The listing builds one solid part. Answer for the finished solid, in the listing's coordinates (mm). A direction names the side the tool comes from. Give positions to 0.01 mm unless a question says otherwise; leave off trailing zeros. Order: outer loops, then holes, each group sorted by start corner. A loop starts at its lowest first (then second) coordinate and runs counter-clockwise, first axis right, second up.
```python
from build123d import *

# Parameters (mm, degrees)
SKETCH1_W                                = 65
SKETCH1_H                                = 38.1
SKETCH1_W_2                              = 41
SKETCH1_H_2                              = 21
BOSS_EXTRUDE1_DEPTH                      = 8
SKETCH2_W                                = 65
SKETCH2_H                                = 38.1
SKETCH2_W_2                              = 59
SKETCH2_H_2                              = 26.1
BOSS_EXTRUDE2_DEPTH                      = 15
F_5_32_0_15625_DIAMETER_HOLE1_D          = 3.96875
F_3_0MM_DOWEL_HOLE1_D                    = 3
F_3_0MM_DOWEL_HOLE1_DEPTH                = 6
CUT_EXTRUDE1_DEPTH                       = 2.25
MIRROR2_AT_THE_SECOND_PLANE_COPY_1_DEPTH = 2.25


with BuildPart() as part:
    # Sketch1 → Boss-Extrude1 (new body)
    with BuildSketch(Plane(origin=(0, 0, 0), x_dir=(0, 0, -1), z_dir=(1, 0, 0))):
        Rectangle(SKETCH1_W, SKETCH1_H)
        Rectangle(SKETCH1_W_2, SKETCH1_H_2, mode=Mode.SUBTRACT)
    extrude(amount=BOSS_EXTRUDE1_DEPTH)

    # Sketch2 → Boss-Extrude2 (add)
    with BuildSketch(Plane(origin=(8, 0, 0), x_dir=(0, 0, -1), z_dir=(1, 0, 0))):
        Rectangle(SKETCH2_W, SKETCH2_H)
        Rectangle(SKETCH2_W_2, SKETCH2_H_2, mode=Mode.SUBTRACT)
    extrude(amount=BOSS_EXTRUDE2_DEPTH)

    # 5/32 (0.15625) Diameter Hole1 (through all)
    with Locations(Plane.ZY):
        with Locations((-23.60854322, 5.122882485), (-23.749, -5.08), (23.749, -5.08), (23.749, 5.08)):
            Hole(F_5_32_0_15625_DIAMETER_HOLE1_D / 2)

    # Ø3.0mm Dowel Hole1
    with Locations(Plane(origin=(0, -13.05, 0), x_dir=(1, 0, 0), z_dir=(0, 1, 0))):
        with Locations((11.5, 25), (11.5, -25)):
            f_3_0mm_dowel_hole1 = Hole(F_3_0MM_DOWEL_HOLE1_D / 2, depth=F_3_0MM_DOWEL_HOLE1_DEPTH)

    # Mirror1: Ø3.0mm Dowel Hole1 across plane
    add(f_3_0mm_dowel_hole1.mirror(Plane.ZX), mode=Mode.SUBTRACT)

    # Sketch7 → Cut-Extrude1 (cut)
    with BuildSketch(Plane(origin=(0, -13.05, 0), x_dir=(1, 0, 0), z_dir=(0, 1, 0))):
        Polygon((8.775, -26.573279484), (11.5, -28.146558967), (14.225, -26.573279484), (14.225, -23.426720516), (11.5, -21.853441033), (8.775, -23.426720516), align=None)
    cut_extrude1 = extrude(amount=-CUT_EXTRUDE1_DEPTH, mode=Mode.SUBTRACT)

    # Mirror2: Cut-Extrude1 across plane
    add(cut_extrude1.mirror(Plane.ZX), mode=Mode.SUBTRACT)

    # Mirror2 at the second plane: Cut-Extrude1 across plane
    add(cut_extrude1.mirror(Plane.XY), mode=Mode.SUBTRACT)

    # Mirror2 at the second plane copy 1 sketc → Mirror2 at the second plane copy 1 (cut)
    with BuildSketch(Plane.XZ.offset(-13.05)):
        Polygon((8.775, -26.573279484), (11.5, -28.146558967), (14.225, -26.573279484), (14.225, -23.426720516), (11.5, -21.853441033), (8.775, -23.426720516), align=None)
    extrude(amount=-MIRROR2_AT_THE_SECOND_PLANE_COPY_1_DEPTH, mode=Mode.SUBTRACT)


solid = part.part
```
1) A tool of negligible diameter and unlimited length cuts with its end or side. For faces 1 (the flat face through (15, -13.05, 0)), 2 (the flat face through (13, 15.3, -26)), 3 (the flat face through (4, 0, -20.5)), from which of +Z, -Z, +X, -X, +Y, -Y can it reach the whole face along a straight path? Write none if from no direction.
Geometry says:
face 1: +X
face 2: none
face 3: +X, -X
2) Find section B-B (z = -17). Write down the section's boundary in (x, y), then the cut area to 3 significant figures.
Geometry says:
outline: (0, -19.05) - (23, -19.05) - (23, -13.05) - (8, -13.05) - (8, -10.5) - (0, -10.5) - close; (0, 10.5) - (8, 10.5) - (8, 13.05) - (23, 13.05) - (23, 19.05) - (0, 19.05) - close
area: 317 mm2
3) Find section A-A (y = 1). Write down the section's boundary in (x, z), then the cut area to 3 significant figures.
Geometry says:
outline: (0, -32.5) - (23, -32.5) - (23, -29.5) - (8, -29.5) - (8, -20.5) - (0, -20.5) - close; (0, 20.5) - (8, 20.5) - (8, 29.5) - (23, 29.5) - (23, 32.5) - (0, 32.5) - close
area: 282 mm2
4) Find section D-D (x = 19.5). Write down the section's boundary in (y, z), then the cut area to 3 significant figures.
Geometry says:
outline: (-19.05, -32.5) - (19.05, -32.5) - (19.05, 32.5) - (-19.05, 32.5) - close; hole (-13.05, -29.5) - (13.05, -29.5) - (13.05, 29.5) - (-13.05, 29.5) - close
area: 937 mm2
5) Straight lines are drawn through the part: probe 1 along Y at (x, z) = (8.25, -7); probe 2 along Y at (x, z) = (4.75, 9.5); probe 3 along Z at (x, y) = (11.5, -16.1). For each, find the intervals that lie inside material, in ascending order.
Geometry says:
probe 1: y = -19.05 to -13.05, 13.05 to 19.05
probe 2: y = -19.05 to -10.5, 10.5 to 19.05
probe 3: z = -32.5 to -26.5, -23.5 to 23.5, 26.5 to 32.5
6) Find section C-C (y = -5.08). Write down the section's boundary in (x, z).
Geometry says:
outline: (0, -32.5) - (23, -32.5) - (23, -29.5) - (8, -29.5) - (8, -25.73) - (0, -25.73) - close; (0, -21.76) - (8, -21.76) - (8, -20.5) - (0, -20.5) - close; (0, 20.5) - (8, 20.5) - (8, 21.76) - (0, 21.76) - close; (0, 25.73) - (8, 25.73) - (8, 29.5) - (23, 29.5) - (23, 32.5) - (0, 32.5) - close
7) For a pull along Z with two mould halves and no side action, classify faces 4 (the flat face through (11, 0, -32.5)), 5 (the flat face through (10.12, 14.16, 27.35)) as +Z half, -Z half, draft (parallel to the pull), parting line (faces both ways), or undercut.
Geometry says:
face 4: -Z half
face 5: undercut
8) Given P1, Ø5, axis at y = -0.5, z = 19.5, coming from the +X side; P2, Ø2.5, axis at y = -5.08, z = 23.749, coming from the -X side, each flat-ended and moving along its own axis, determine where each tip first touches the part or whether it passes through.
Geometry says:
P1: stops at x = 8
P2: passes through
